Part model, mm, in its own coordinate system. Give positions to 0.01 mm unless a question says otherwise; leave off trailing zeros. Order: outer loops, then holes, each group sorted by start corner. A loop starts at its lowest first (then second) coordinate and runs counter-clockwise, first axis right, second up.
1. Drop flat-ended pins along their axis: pin 1 Ø7.5 at (y, z) = (57.15, -115.96) entering from -X; pin 2 Ø2.5 at (x, z) = (-4.94, 17.39) entering from +Y. Give the stop position or say it passes through.
2. Slice it at C-C on y = 38.5. List the corners of the cut face in (x, z), and give its area (3 significant figures).
3. Probe line 1 (Z direction, x = -14.5, y = 61.5); line 2 (X direction, y = 22.5, z = -136.5); line 3 (X direction, y = 50, z = 16). List the from-to ranges inside material, lowest first.
4. Slice it at A-A on x = -14.5. Give the number of separate pieces and of enclosed holes in the cut face, and give its area (3 significant figures).
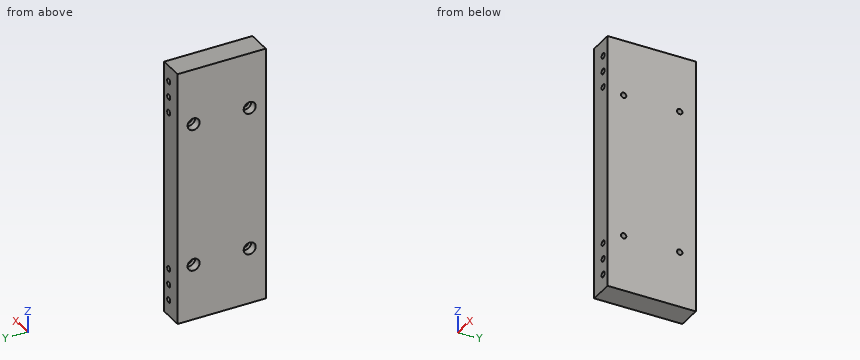
Autodesk Inventor part; units mm, degrees
ref_plane "YZ Plane" through (0, 0, 0) normal (1, 0, 0) x (0, 1, 0)
ref_plane "XZ Plane" through (0, 0, 0) normal (0, 1, 0) x (-1, 0, 0)
ref_plane "XY Plane" through (0, 0, 0) normal (0, 0, 1) x (1, 0, 0)
sketch "Sketch1" plane through (0, 0, 0) normal (0, 1, 0) x (-1, 0, 0)
  line L0 (17.6389, 42.7869) -> (-1.4111, 42.7869)
  line L1 (-1.4111, 42.7869) -> (-1.4111, -160.4131)
  line L2 (-1.4111, -160.4131) -> (17.6389, -160.4131)
  line L3 (17.6389, -160.4131) -> (17.6389, 42.7869)
  point P0 (0, 0)
  dimension "d0" = 19.05
  dimension "d1" = 203.2
extrude "Extrusion1" add sketch "Sketch1" along normal blind 69.85
sketch "Sketch2" plane through (0, 69.85, 0) normal (0, 1, 0) x (1, 0, 0)
  line L0 (-17.6389, -42.7869) -> (1.4111, -42.7869)
  line L1 (1.4111, -42.7869) -> (1.4111, 160.4131)
  line L2 (1.4111, 160.4131) -> (-17.6389, 160.4131)
  point P0 (0, 0)
  point P1 (-4.9389, -30.0869)
  point P2 (-4.9389, -17.3869)
  point P3 (-4.9389, -4.6869)
  point P4 (-4.9389, 135.0131)
  point P5 (-4.9389, 122.3131)
  point P6 (-4.9389, 147.7131)
  dimension "d4" = 0
  dimension "d5" = 0
  dimension "d6" = 12.7
  dimension "d7" = 12.7
  dimension "d8" = 12.7
  dimension "d9" = 6.35
  dimension "d10" = 12.7
  dimension "d11" = 6.35
  dimension "d12" = 0
  dimension "d13" = 12.7
  dimension "d14" = 12.7
  dimension "d15" = 0
hole "Hole1" at (-4.9389, 69.85, 30.0869) at (-4.9389, 69.85, 17.3869) at (-4.9389, 69.85, 4.6869) at (-4.9389, 69.85, -135.0131) at (-4.9389, 69.85, -122.3131) at (-4.9389, 69.85, -147.7131) direction (0, -1, 0) diameter 4.318 end through all
sketch "Sketch3" plane through (-17.6389, 0, -160.4131) normal (-1, 0, 0) x (0, 0, 1)
  line L0 (101.6, 78.5929) -> (101.6, -10.5439)
  line L1 (0, 0) -> (0, 69.85)
  line L2 (203.2, 0) -> (0, 0)
  line L3 (0, 69.85) -> (203.2, 69.85)
  point P0 (160.4131, 0)
  point P1 (44.45, 57.15)
  point P2 (44.45, 12.7)
  point P3 (158.75, 57.15)
  point P4 (158.75, 12.7)
  dimension "d23" = 101.6
  dimension "d24" = 0
  dimension "d25" = 12.7
  dimension "d26" = 12.7
  dimension "d27" = 57.15
  dimension "d28" = 0
  dimension "d29" = 0
  dimension "d30" = 0
  dimension "d31" = 57.15
hole "Hole2" at (-17.6389, 57.15, -115.9631) at (-17.6389, 12.7, -115.9631) at (-17.6389, 57.15, -1.6631) at (-17.6389, 12.7, -1.6631) direction (1, 0, 0) diameter 4.318 depth 25.4 tip angle 118 counterbore diameter 9.525 counterbore depth 6.35
properties part number "BackBatteryPlate"
Data:
1. pin 1: stops at x = -11.29
1. pin 2: passes through
2. outline: (-17.64, -160.41) - (1.41, -160.41) - (1.41, 42.79) - (-17.64, 42.79) - close; hole circle Ø4.32 at (-4.94, -147.71); hole circle Ø4.32 at (-4.94, -135.01); hole circle Ø4.32 at (-4.94, -122.31); hole circle Ø4.32 at (-4.94, 4.69); hole circle Ø4.32 at (-4.94, 17.39); hole circle Ø4.32 at (-4.94, 30.09)
2. area: 3,780 mm2
3. line 1: z = -160.41 to -117.9, -114.02 to -3.6, 0.28 to 42.79
3. line 2: x = -17.64 to -6.5, -3.37 to 1.41
3. line 3: x = -17.64 to -6.59, -3.28 to 1.41
4. separate pieces: 1
4. enclosed holes: 4
4. area: 13,900 mm2
